Verification items for the finished model (mm, model axes). A direction names the side the tool comes from. Coordinates: 2 decimals unless noted, no trailing zeros. Write each loop counter-clockwise with the first axis right and the second up, starting at its lowest first coordinate (ties: lowest second). Pieces come first, ordered by that corner, then holes. Notation, with made-up numbers: (-3, 49.5) - (53, 49.5) arc R13 cw to (53, 56.5) - close; hole circle Ø1 at (36.5, -2.75). An arc over 180 degrees is marked (long way). Answer as CSV lines item,"result". Start each with the question number.
```python
from build123d import *

# Parameters (mm, degrees)
F0_W     = 1447.8
F0_H     = 406.4
F6_DEPTH = 12.7
F1_R     = 9.525
F1_R_2   = 6.35
F7_DEPTH = 180.975
F5_R     = 9.525
F5_R_2   = 6.35
F8_DEPTH = 361.95
F4_R     = 12.7
F4_R_2   = 6.35
F9_DEPTH = 361.95


with BuildPart() as f6:
    # F0 (on Top) → F6 (new body, symmetric)
    with BuildSketch(Plane.XY):
        Rectangle(F0_W, F0_H)
    extrude(amount=F6_DEPTH, both=True)

    # F1 (on Right) → F7 (join, symmetric)
    with BuildSketch(Plane.YZ):
        with Locations((-210.82, 0)):
            Circle(F1_R)
        with Locations((-210.82, 0)):
            Circle(F1_R_2, mode=Mode.SUBTRACT)
    extrude(amount=F7_DEPTH, both=True)

    # F5 (on offset) → F8 (join)
    with BuildSketch(Plane.YZ.offset(361.95)):
        with Locations((210.82, 0)):
            Circle(F5_R)
        with Locations((210.82, 0)):
            Circle(F5_R_2, mode=Mode.SUBTRACT)
    extrude(amount=F8_DEPTH)

    # F4 (on offset) → F9 (join)
    with BuildSketch(Plane.YZ.offset(-361.696)):
        with Locations((210.82, 0)):
            Circle(F4_R)
        with Locations((210.82, 0)):
            Circle(F4_R_2, mode=Mode.SUBTRACT)
    extrude(amount=-F9_DEPTH)


solid = f6.part
```
1. Cross-section at B-B (z = 0). Record the cut outline in (x, y) (3 decimals).
2. Depth check by flat-ended pin: P1, Ø1, axis at x = -69, z = -5.5, coming from the +Y side; P2, Ø14.5, axis at y = 210.82, z = 0, coming from the +X side; P3, Ø10, axis at x = 32.5, z = 8.5, coming from the -Y side; P4, Ø8.5, axis at y = 214.5, z = 3, coming from the -X side. Enter the tip coordinate at first touch or a pass-through.
3. Scan lines: line 1 along Z through (x, y) = (13.5, -210.82) (3 decimals); line 2 along Y through (x, z) = (-305, 4); line 3 along Y through (x, z) = (-127, 7.75). Record each from-to range of solid material in increasing order. Write a range as from..to.
4. Cross-section at C-C (x = -160.5). Record the cut outline in (y, z) (3 decimals), and give its area (3 significant figures).
5. Cross-section at D-D (x = 336.5). Record the cut outline in (y, z).
6. Draft check along Y on faces 3 (the face through (-723.9, -3, 0)), 4 (the face through (-10, 203.2, 0)). Enter one of: pulls with the +Y half, pulls with the -Y half, needs draft (parallel to the pull), parting line crosses it, or undercut.
7. Access from +Z, -Z, +X, -X, +Y, -Y to the whole of each face (thin tool, end or side, straight path). Record for faces 1 (the face through (723.9, 6, 0)), 2 (the face through (-10, -203.2, 6)).
8. Cross-section at A-A (x = -619). Record the cut outline in (y, z).
Completed:
1,outline,"(-723.9, -203.2) - (-180.975, -203.2) - (-180.975, -204.47) - (180.975, -204.47) - (180.975, -203.2) - (723.9, -203.2) - (723.9, 204.47) - (361.95, 204.47) - (361.95, 203.2) - (-361.696, 203.2) - (-361.696, 204.47) - (-723.646, 204.47) - (-723.646, 203.2) - (-723.9, 203.2) - close; (-723.646, 217.17) - (-361.696, 217.17) - (-361.696, 223.52) - (-723.646, 223.52) - close; (-180.975, -220.345) - (180.975, -220.345) - (180.975, -217.17) - (-180.975, -217.17) - close; (361.95, 217.17) - (723.9, 217.17) - (723.9, 220.345) - (361.95, 220.345) - close"
2,P1,"stops at y = 203.2"
2,P2,"stops at x = 723.9"
2,P3,"stops at y = -219.68"
2,P4,"stops at x = -723.65"
3,line 1,"z = -9.525..-6.35, 6.35..9.525"
3,line 2,"y = -203.2..203.2"
3,line 3,"y = -216.36..-205.28, -203.2..203.2"
4,outline,"(-203.2, -12.7) - (203.2, -12.7) - (203.2, 12.7) - (-203.2, 12.7) - (-203.2, 5.715) arc R9.525 ccw (long way) to (-203.2, -5.715) - close; hole circle Ø12.7 at (-210.82, 0)"
4,area,"10,500 mm2"
5,outline,"(-203.2, -12.7) - (203.2, -12.7) - (203.2, 12.7) - (-203.2, 12.7) - close"
6,face 3,"needs draft"
6,face 4,"undercut"
7,face 1,"+Z, -Z, +X, +Y, -Y"
7,face 2,"none"
8,outline,"(-203.2, -12.7) - (203.2, -12.7) - (203.2, -10.16) arc R12.7 ccw (long way) to (203.2, 10.16) - (203.2, 12.7) - (-203.2, 12.7) - close; hole circle Ø12.7 at (210.82, 0)"
